```python
from build123d import *

# Parameters (mm, degrees)
SKETCH1_W           = 26
SKETCH1_H           = 26
SKETCH1_R           = 1.7
BOSS_EXTRUDE1_DEPTH = 1.6
SKETCH2_W           = 6
SKETCH2_H           = 4.29
BOSS_EXTRUDE2_DEPTH = 3
SKETCH3_W           = 2.5
SKETCH3_H           = 15.5
BOSS_EXTRUDE3_DEPTH = 2.5
SKETCH4_W           = 3
SKETCH4_H           = 3
BOSS_EXTRUDE4_DEPTH = 1


with BuildPart() as part:
    # Sketch1 → Boss-Extrude1 (new body)
    with BuildSketch(Plane(origin=(0, 0, 0), x_dir=(1, 0, 0), z_dir=(0, 1, 0))):
        Rectangle(SKETCH1_W, SKETCH1_H)
        with Locations(Location((-10.3, 10.3, 0), (0, 0, 270))):
            Circle(SKETCH1_R, mode=Mode.SUBTRACT)
        with Locations(Location((10.3, 10.3, 0), (0, 0, 270))):
            Circle(SKETCH1_R, mode=Mode.SUBTRACT)
        with Locations(Location((-10.3, -10.3, 0), (0, 0, 270))):
            Circle(SKETCH1_R, mode=Mode.SUBTRACT)
        with Locations(Location((10.3, -10.3, 0), (0, 0, 270))):
            Circle(SKETCH1_R, mode=Mode.SUBTRACT)
    extrude(amount=BOSS_EXTRUDE1_DEPTH)

    # Sketch2 → Boss-Extrude2 (add)
    with BuildSketch(Plane(origin=(0, 1.6, 0), x_dir=(1, 0, 0), z_dir=(0, 1, 0))):
        with Locations((0, 9.955)):
            Rectangle(SKETCH2_W, SKETCH2_H)
        with Locations((0, -9.955)):
            Rectangle(SKETCH2_W, SKETCH2_H)
    extrude(amount=BOSS_EXTRUDE2_DEPTH)

    # Sketch3 → Boss-Extrude3 (add)
    with BuildSketch(Plane.XZ):
        with Locations((-11.65, 0)):
            Rectangle(SKETCH3_W, SKETCH3_H)
        with Locations((11.65, 0)):
            Rectangle(SKETCH3_W, SKETCH3_H)
    extrude(amount=BOSS_EXTRUDE3_DEPTH)

    # Sketch4 → Boss-Extrude4 (add)
    with BuildSketch(Plane(origin=(0, 1.6, 0), x_dir=(1, 0, 0), z_dir=(0, 1, 0))):
        Rectangle(SKETCH4_W, SKETCH4_H)
    extrude(amount=BOSS_EXTRUDE4_DEPTH)


solid = part.part
```
Verification items for the finished model (mm, model axes). A direction names the side the tool comes from. Round coordinates to 2 decimals unless told otherwise and drop trailing zeros. Loops run counter-clockwise (first coordinate to the right, second up) from the corner with the lowest first, then second, coordinate; pieces in that order, holes last. Notation, with made-up numbers: (-21, 89.5) -> (19, 89.5) arc R29 cw to (19, 120.5) -> close; hole circle Ø1 at (-25, 9.25). An arc over 180 degrees is marked (long way). Answer as a JSON object with one key per item and string values.
Q1. Section check B-B (z = 10.3). Record the boundary of the cut face in (x, y).
Data:
{"outline": "(-13, 0) -> (-12, 0) -> (-12, 1.6) -> (-13, 1.6) -> close; (-8.6, 0) -> (8.6, 0) -> (8.6, 1.6) -> (3, 1.6) -> (3, 4.6) -> (-3, 4.6) -> (-3, 1.6) -> (-8.6, 1.6) -> close; (12, 0) -> (13, 0) -> (13, 1.6) -> (12, 1.6) -> close"}
Q2. Scan lines: line 1 (X direction, y = 0.7, z = 10.3); line 2 (X direction, y = -1, z = -0.25); line 3 (Z direction, x = -2.75, y = 4.25). Record each from-to range of solid material in increasing order. Write a range as from..to.
Data:
{"line 1": "x = -13..-12, -8.6..8.6, 12..13", "line 2": "x = -12.9..-10.4, 10.4..12.9", "line 3": "z = -12.1..-7.81, 7.81..12.1"}
Q3. Section check C-C (x = -2). Record the boundary of the cut face in (y, z).
Data:
{"outline": "(0, -13) -> (1.6, -13) -> (1.6, -12.1) -> (4.6, -12.1) -> (4.6, -7.81) -> (1.6, -7.81) -> (1.6, 7.81) -> (4.6, 7.81) -> (4.6, 12.1) -> (1.6, 12.1) -> (1.6, 13) -> (0, 13) -> close"}
Q4. Section check D-D (z = 3.5). Record the boundary of the cut face in (x, y), then the cut area to 3 significant figures.
Data:
{"outline": "(-13, 0) -> (-12.9, 0) -> (-12.9, -2.5) -> (-10.4, -2.5) -> (-10.4, 0) -> (10.4, 0) -> (10.4, -2.5) -> (12.9, -2.5) -> (12.9, 0) -> (13, 0) -> (13, 1.6) -> (-13, 1.6) -> close", "area": "54.1 mm2"}
Q5. Go/stop test with flat-tipped pins: P1, Ø0.8, axis at y = -1.5, z = -1.5, coming from the -X side; P2, Ø1.2, axis at x = 11, y = -1, coming from the +Z side; P3, Ø0.9, axis at x = -0.5, y = 2.5, coming from the +Z side. Record where each tip stops, or that it passes through.
Data:
{"P1": "stops at x = -12.9", "P2": "stops at z = 7.75", "P3": "stops at z = 12.1"}
Q6. Section check A-A (y = 4.25). Record the boundary of the cut face in (x, z).
Data:
{"outline": "(-3, -12.1) -> (3, -12.1) -> (3, -7.81) -> (-3, -7.81) -> close; (-3, 7.81) -> (3, 7.81) -> (3, 12.1) -> (-3, 12.1) -> close"}
Q7. Access from +Z, -Z, +X, -X, +Y, -Y to the whole of each face (thin tool, end or side, straight path). Record for faces 4 (the flat face through (0, 3, -12.1)), 5 (the flat face through (0, 2, 1.5)), 6 (the flat face through (3, 3, 10)), 7 (the flat face through (10.4, -1, 0)).
Data:
{"face 4": "-Z, +X, -X, +Y", "face 5": "+X, -X, +Y", "face 6": "+Z, -Z, +X, +Y", "face 7": "+Z, -Z, -Y"}
Q8. Draft check along Z on faces 1 (the flat face through (0, 3, -7.81)), 2 (the flat face through (0, 4.6, 10)), 3 (the flat face through (0, 1, -13)). Enter one of: pulls with the +Z half, pulls with the -Z half, needs draft (parallel to the pull), parting line crosses it, or undercut.
Data:
{"face 1": "undercut", "face 2": "needs draft", "face 3": "pulls with the -Z half"}
